from build123d import *

# Parameters (mm, degrees)
SKETCH2_W               = 47.498
SKETCH2_H               = 13.9954
BOSS_EXTRUDE1_DEPTH     = 9.0043
SKETCH3_R               = 3.01244
SKETCH3_R_2             = 3.5052
CUT_EXTRUDE1_DEPTH      = 7.9977
CUT_EXTRUDE1_DEPTH_BACK = 7.9977
SKETCH5_OUTSIDE_W       = 60.036
SKETCH5_OUTSIDE_H       = 30.546
CUT_EXTRUDE2_DEPTH      = 7.9977
CUT_EXTRUDE2_DEPTH_BACK = 7.9977
CUT_EXTRUDE3_DEPTH      = 7.9977
CUT_EXTRUDE3_DEPTH_BACK = 7.9977
FILLET1_R               = 4.7752
SKETCH7_W               = 11.5062
SKETCH7_H               = 8.1026
CUT_EXTRUDE4_DEPTH      = 10.0043
CUT_EXTRUDE4_DEPTH_BACK = 10.0043


with BuildPart() as part:
    # Sketch2 → Boss-Extrude1 (new body, symmetric)
    with BuildSketch(Plane(origin=(0, 0, 0), x_dir=(1, 0, 0), z_dir=(0, 1, 0))):
        Rectangle(SKETCH2_W, SKETCH2_H)
    extrude(amount=BOSS_EXTRUDE1_DEPTH, both=True)

    # Sketch3 → Cut-Extrude1 (cut, two sides)
    with BuildSketch(Plane.XY) as cut_extrude1_sk:
        with Locations((18.7452, -1.9939)):
            Circle(SKETCH3_R)
        with Locations((0.4826, 1.9939)):
            Circle(SKETCH3_R_2)
    extrude(amount=CUT_EXTRUDE1_DEPTH, mode=Mode.SUBTRACT)
    extrude(cut_extrude1_sk.sketch, amount=-CUT_EXTRUDE1_DEPTH_BACK, mode=Mode.SUBTRACT)

    # Sketch5 outside → Cut-Extrude2 (cut, two sides)
    with BuildSketch(Plane.XY) as cut_extrude2_sk:
        Rectangle(SKETCH5_OUTSIDE_W, SKETCH5_OUTSIDE_H)
        with BuildLine():
            Line((16.610431019, -9.0043), (21.2471, -6.327317915))
            ThreePointArc((21.2471, -6.327317915), (23.078617915, -4.4958), (23.749, -1.9939))
            Line((23.749, -1.9939), (23.749, -1.317979314))
            ThreePointArc((23.749, -1.317979314), (23.056619993, 1.221641146), (21.171090378, 3.058442776))
            Line((21.171090378, 3.058442776), (10.44448, 9.0043))
            Line((10.44448, 9.0043), (-1.0414, 9.0043))
            Line((-1.0414, 9.0043), (-23.749, -1.584427778))
            Line((-23.749, -1.584427778), (-23.749, -9.0043))
            Line((-23.749, -9.0043), (16.610431019, -9.0043))
        make_face(mode=Mode.SUBTRACT)
    extrude(amount=CUT_EXTRUDE2_DEPTH, mode=Mode.SUBTRACT)
    extrude(cut_extrude2_sk.sketch, amount=-CUT_EXTRUDE2_DEPTH_BACK, mode=Mode.SUBTRACT)

    # Sketch6 → Cut-Extrude3 (cut, two sides)
    with BuildSketch(Plane.XY) as cut_extrude3_sk:
        with BuildLine():
            Line((-1.524, -9.0043), (-5.5118, -5.0165))
            Line((-5.5118, -5.0165), (-13.629006931, -5.0165))
            ThreePointArc((-13.629006931, -5.0165), (-18.655709059, -7.50508415), (-23.749, -5.155792182))
            Line((-23.749, -5.155792182), (-23.749, -9.0043))
            Line((-23.749, -9.0043), (-1.524, -9.0043))
        make_face()
    extrude(amount=CUT_EXTRUDE3_DEPTH, mode=Mode.SUBTRACT)
    extrude(cut_extrude3_sk.sketch, amount=-CUT_EXTRUDE3_DEPTH_BACK, mode=Mode.SUBTRACT)

    # Fillet1
    fillet1_edges = [part.edges().sort_by_distance(p)[0] for p in [
        (-13.629006931, -5.0165, 0),
        (-5.5118, -5.0165, 0),
        (-1.524, -9.0043, 0),
    ]]
    fillet(fillet1_edges, radius=FILLET1_R)

    # Sketch7 → Cut-Extrude4 (cut, two sides)
    with BuildSketch(Plane(origin=(0, 0, 0), x_dir=(1, 0, 0), z_dir=(0, 1, 0))) as cut_extrude4_sk:
        with Locations((17.9959, 0)):
            Rectangle(SKETCH7_W, SKETCH7_H)
    extrude(amount=CUT_EXTRUDE4_DEPTH, mode=Mode.SUBTRACT)
    extrude(cut_extrude4_sk.sketch, amount=-CUT_EXTRUDE4_DEPTH_BACK, mode=Mode.SUBTRACT)


solid = part.part
Part model, mm, in its own coordinate system. A direction names the side the tool comes from. Coordinates: 2 decimals unless noted, no trailing zeros. Order: outer loops, then holes, each group sorted by start corner. A loop starts at its lowest first (then second) coordinate and runs counter-clockwise, first axis right, second up.
(1) Pull direction X, two halves, no side cores. Call faces 4 (the face through (23.06, -4.53, -5.55)), 5 (the face through (-13.24, -5.28, 0.1)), 6 (the face through (8, -9.004, 0)): pulls with the +X half, pulls with the -X half, needs draft (parallel to the pull), parting line crosses it, or undercut.
Check sheet entries:
face 4: pulls with the +X half
face 5: undercut
face 6: needs draft
(2) Tool access for faces 1 (the face through (-10, -5.016, 0)), 2 (the face through (15, 0, 4.051)), 3 (the face through (15.736, -1.861, 5.545)): list every direction of +Z, -Z, +X, -X, +Y, -Y with a clear straight run to the whole face (end or side of a thin tool).
Check sheet entries:
face 1: +Z, -Z, -Y
face 2: +X, +Y, -Y
face 3: +Z, -Z
(3) Slice it at C-C, the plane y = -0.25. Write the cut outline in (x, z), and give its area (3 significant figures).
Check sheet entries:
outline: (-20.89, -7) - (-2.21, -7) - (-2.21, 7) - (-20.89, 7) - close; (3.18, -7) - (16.29, -7) - (16.29, -4.05) - (12.24, -4.05) - (12.24, 4.05) - (16.29, 4.05) - (16.29, 7) - (3.18, 7) - close; (21.2, -7) - (23.63, -7) - (23.63, -4.05) - (21.2, -4.05) - close; (21.2, 4.05) - (23.63, 4.05) - (23.63, 7) - (21.2, 7) - close
area: 426 mm2
(4) Probe L1, parallel to X at y = -0.75, z = -4.75; L2, parallel to X at y = 1.5, z = 5.75; L3, parallel to X at y = 3.5, z = 2. List the from-to ranges inside material, lowest first.
Check sheet entries:
L1: x = -21.96 to -1.7, 2.66 to 16, 21.49 to 23.72
L2: x = -17.13 to -2.99, 3.95 to 22.88
L3: x = -12.85 to -2.68, 3.65 to 12.24
(5) Slice it at A-A, the plane y = -3. Write the cut outline in (x, z), and give its area (3 significant figures).
Check sheet entries:
outline: (-23.75, -7) - (15.91, -7) - (15.91, -4.05) - (12.24, -4.05) - (12.24, 4.05) - (15.91, 4.05) - (15.91, 7) - (-23.75, 7) - close; (21.58, -7) - (23.65, -7) - (23.65, -4.05) - (21.58, -4.05) - close; (21.58, 4.05) - (23.65, 4.05) - (23.65, 7) - (21.58, 7) - close
area: 537 mm2
(6) Pin check, flat tips, straight feed: pin 1 Ø1.3 at (x, z) = (-9, 1.5) entering from -Y; pin 2 Ø1.5 at (y, z) = (6, -2.5) entering from -X; pin 3 Ø2.5 at (y, z) = (-3.5, -1) entering from +X. Stop position of each tip, or through.
Check sheet entries:
pin 1: stops at y = -5.02
pin 2: stops at x = -9.09
pin 3: stops at x = 12.24
(7) Slice it at B-B, the plane x = 19. Write the cut outline in (y, z), and give its area (3 significant figures).
Check sheet entries:
outline: (-7.62, -7) - (-5, -7) - (-5, -4.05) - (-7.62, -4.05) - close; (-7.62, 4.05) - (-5, 4.05) - (-5, 7) - (-7.62, 7) - close; (1.01, -7) - (4.26, -7) - (4.26, -4.05) - (1.01, -4.05) - close; (1.01, 4.05) - (4.26, 4.05) - (4.26, 7) - (1.01, 7) - close
area: 34.7 mm2
(8) Slice it at D-D, the plane z = 2.75. Write the cut outline in (x, y), and give its area (3 significant figures).
Check sheet entries:
outline: (-23.75, -5.16) arc R6.5 ccw to (-14.67, -6.07) arc R4.78 cw to (-11.68, -5.02) - (-7.49, -5.02) arc R4.78 cw to (-4.11, -6.42) - (-2.92, -7.61) arc R4.78 ccw to (0.45, -9) - (12.24, -9) - (12.24, 8.01) - (10.44, 9) - (-1.04, 9) - (-23.75, -1.58) - close; hole circle Ø7.01 at (0.48, 1.99)
area: 426 mm2
